from build123d import *

# Parameters (mm, degrees)
F1_DEPTH  = 25.4
F2_T      = -6.35
F4_DEPTH  = 25.4
F4_TAPER  = 4
F6_DEPTH  = 25.4
F6_TAPER  = 4
F8_DEPTH  = 25.4
F8_TAPER  = 4
F10_DEPTH = 25.4
F10_TAPER = 4


with BuildPart() as f1:
    # F0 (on Top) → F1 (new body)
    with BuildSketch(Plane.XY):
        Polygon((-50.552804023, 67.5352037176), (-50.552804023, -59.4647962824), (74.7760616566, -61.1142246816), (76.4363430164, 65.8749223579), align=None)
    extrude(amount=F1_DEPTH)

    # F2
    f2_openings = [f1.faces().sort_by_distance(p)[0] for p in [
        (12.528514, 3.347032, 25.4),
    ]]
    offset(amount=F2_T, openings=f2_openings)

    # F3 (on face) → F4 (join)
    with BuildSketch(Plane.XY.offset(6.35)):
        Polygon((57.2176291898, 52.4085088478), (57.1761186085, 49.2335088478), (59.3918302252, 46.959092404), (62.5668302252, 46.9175818226), (64.841246669, 49.1332934393), (64.8827572503, 52.3082934393), (62.6670456336, 54.5827098831), (59.4920456336, 54.6242204645), align=None)
    extrude(amount=F4_DEPTH, taper=F4_TAPER)

    # F5 (on face) → F6 (join)
    with BuildSketch(Plane.XY.offset(6.35)):
        Polygon((-38.6233556014, -41.3551133633), (-38.6233556014, -44.5301133633), (-36.3782915711, -46.7751773935), (-33.2032915711, -46.7751773935), (-30.9582275409, -44.5301133633), (-30.9582275409, -41.3551133633), (-33.2032915711, -39.110049333), (-36.3782915711, -39.110049333), align=None)
    extrude(amount=F6_DEPTH, taper=F6_TAPER)

    # F7 (on face) → F8 (join)
    with BuildSketch(Plane.XY.offset(6.35)):
        Polygon((60.750235939, -40.5762630585), (57.575235939, -40.5762630585), (55.3301719088, -42.8213270888), (55.3301719088, -45.9963270888), (57.575235939, -48.241391119), (60.750235939, -48.241391119), (62.9952999693, -45.9963270888), (62.9952999693, -42.8213270888), align=None)
    extrude(amount=F8_DEPTH, taper=F8_TAPER)

    # F9 (on face) → F10 (join)
    with BuildSketch(Plane.XY.offset(6.35)):
        Polygon((64.0322734141, 31.7149339752), (61.6480793024, 33.811656045), (58.4795930846, 33.6083826148), (56.3828710148, 31.2241885032), (56.586144445, 28.0557022853), (58.9703385566, 25.9589802155), (62.1388247745, 26.1622536457), (64.2355468443, 28.5464477573), align=None)
    extrude(amount=F10_DEPTH, taper=F10_TAPER)


solid = f1.part
Design review of the part built by this model. Coordinates are the model's own, in mm. Coordinates: 2 decimals unless noted, no trailing zeros. Order: outer loops, then holes, each group sorted by start corner. A loop starts at its lowest first (then second) coordinate and runs counter-clockwise, first axis right, second up. Notation, with made-up numbers: M 70,53.5 L 86,53.5 A17 ccw 86,58.5 Z; hole C -4.75,31 d10. An arc over 180 degrees is marked long. Use a Markdown table: item, result.
(1) Add section A-A (z = 29.5). Count the separate pieces of the cut face and the enclosed holes in it, then the cut area to 3 significant figures.
Worked answers:
| item | result |
|---|---|
| separate pieces | 4 |
| enclosed holes | 0 |
| area | 65.0 mm2 |
(2) For P1, Ø4, axis at x = 49.5, y = 2.5, coming from the +Z side; P2, Ø2, axis at x = 26, z = 3.5, coming from the -Y side; P3, Ø4, axis at x = 47.5, z = 21.5, coming from the +Y side, all flat-tipped, find the tip position at first contact; note any pin that passes through.
Worked answers:
| item | result |
|---|---|
| P1 | stops at z = 6.35 |
| P2 | stops at y = -60.49 |
| P3 | stops at y = 66.28 |
(3) Draft analysis for pull direction X (two halves, no side actions). For faces 1 (the flat face through (63.11, 48.67, 18.87)), 2 (the flat face through (12, 4, 0)), state which applies: released by +X, released by -X, zero draft, split by the parting line, or undercut.
Worked answers:
| item | result |
|---|---|
| face 1 | undercut |
| face 2 | zero draft |
(4) Add section D-D (x = 36). Give the boundary of the cut face in (y, z).
Worked answers:
| item | result |
|---|---|
| outline | M -60.6,0 L 66.4,0 L 66.4,25.4 L 60.05,25.4 L 60.05,6.35 L -54.25,6.35 L -54.25,25.4 L -60.6,25.4 Z |
(5) Wall thickness on probe 1 along Y at (x, z) = (62, 12.5); probe 2 along Z at (x, y) = (-8, -52): over which ranges is each line inside the solid? List them lowest first.
Worked answers:
| item | result |
|---|---|
| probe 1 | y = -60.95 to -54.6, -46.38 to -42.43, 26.66 to 32.93, 47.36 to 54.16, 59.71 to 66.06 |
| probe 2 | z = 0 to 6.35 |
(6) Add section B-B (y = -37). Give the boundary of the cut face in (x, z).
Worked answers:
| item | result |
|---|---|
| outline | M -50.55,0 L 75.09,0 L 75.09,25.4 L 68.74,25.4 L 68.74,6.35 L -44.2,6.35 L -44.2,25.4 L -50.55,25.4 Z |
